from build123d import *

# Parameters (mm, degrees)
SKETCH1_W           = 28
SKETCH1_H           = 48
BOSS_EXTRUDE3_DEPTH = 60
SKETCH6_W           = 10
SKETCH6_H           = 35
CUT_EXTRUDE7_DEPTH  = 48
SKETCH7_W           = 25
SKETCH7_H           = 10
CUT_EXTRUDE8_DEPTH  = 48
SKETCH8_W           = 35
SKETCH8_H           = 28
BOSS_EXTRUDE4_DEPTH = 92
SKETCH9_R           = 6.25
CUT_EXTRUDE9_DEPTH  = 59
CUT_EXTRUDE12_DEPTH = 59
CUT_EXTRUDE13_DEPTH = 59
CUT_EXTRUDE18_DEPTH = 11


with BuildPart() as part:
    # Sketch1 → Boss-Extrude3 (new body)
    with BuildSketch(Plane.XY):
        with Locations((14, 24)):
            Rectangle(SKETCH1_W, SKETCH1_H)
    extrude(amount=BOSS_EXTRUDE3_DEPTH)

    # Sketch6 → Cut-Extrude7 (cut)
    with BuildSketch(Plane(origin=(0, 48, 0), x_dir=(1, 0, 0), z_dir=(0, 1, 0))):
        with Locations((23, -30)):
            Rectangle(SKETCH6_W, SKETCH6_H)
    extrude(amount=-CUT_EXTRUDE7_DEPTH, mode=Mode.SUBTRACT)

    # Sketch7 → Cut-Extrude8 (cut)
    with BuildSketch(Plane.ZY):
        with Locations((30, 43)):
            Rectangle(SKETCH7_W, SKETCH7_H)
    extrude(amount=-CUT_EXTRUDE8_DEPTH, mode=Mode.SUBTRACT)

    # Sketch8 → Boss-Extrude4 (add)
    with BuildSketch(Plane.ZY):
        with Locations((30, 14)):
            Rectangle(SKETCH8_W, SKETCH8_H)
    extrude(amount=BOSS_EXTRUDE4_DEPTH)

    # Sketch9 → Cut-Extrude9 (cut)
    with BuildSketch(Plane.XY.offset(47.5)):
        with Locations((-35, 14)):
            Circle(SKETCH9_R)
    extrude(amount=-CUT_EXTRUDE9_DEPTH, mode=Mode.SUBTRACT)

    # Sketch16 → Cut-Extrude12 (cut)
    with BuildSketch(Plane(origin=(0, 28, 0), x_dir=(1, 0, 0), z_dir=(0, 1, 0))):
        Polygon((-92, -30), (-73.408450704, -12.5), (-92, -12.5), align=None)
    extrude(amount=-CUT_EXTRUDE12_DEPTH, mode=Mode.SUBTRACT)

    # Sketch17 → Cut-Extrude13 (cut)
    with BuildSketch(Plane(origin=(0, 28, 0), x_dir=(1, 0, 0), z_dir=(0, 1, 0))):
        Polygon((-92, -30), (-92, -47.5), (-74.705382998, -47.5), align=None)
    extrude(amount=-CUT_EXTRUDE13_DEPTH, mode=Mode.SUBTRACT)

    # Sketch18 → Cut-Extrude18 (cut)
    with BuildSketch(Plane(origin=(0, 28, 0), x_dir=(1, 0, 0), z_dir=(0, 1, 0))):
        Polygon((-92, -30), (-78.644507081, -43.514096673), (-78.164969417, -16.977253409), align=None)
    extrude(amount=-CUT_EXTRUDE18_DEPTH, mode=Mode.SUBTRACT)


solid = part.part
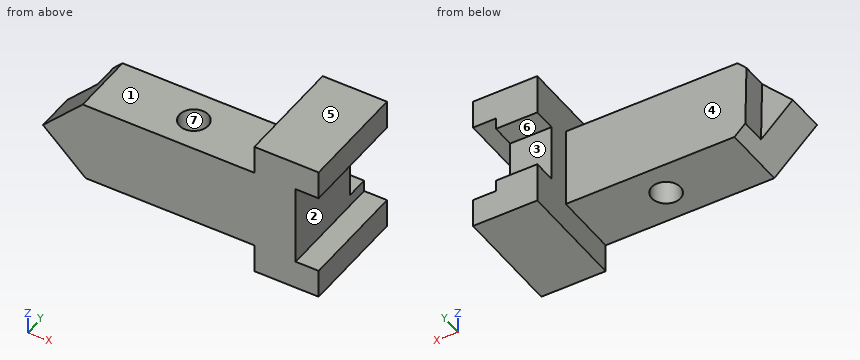
Could you check a few things on this model? Use its own coordinates, in mm. Face numbers are marked on the shaded views. A direction names the side the tool comes from. Give positions to 0.01 mm unless a question says otherwise; leave off trailing zeros. Order: outer loops, then holes, each group sorted by start corner. A loop starts at its lowest first (then second) coordinate and runs counter-clockwise, first axis right, second up. Notation, with made-up numbers: (39, 53) - (50, 53) arc R14 cw to (50, 65) - close; hole circle Ø1 at (-1, -15.5). An arc over 180 degrees is marked (long way). Return JSON: item names as keys, results as strings. Group by question number.
Q1. Suppose I cut it at C-C, the plane y = 23. Please give me the cut outline in (x, z), and give its area (3 significant figures).
Q2. Which directions (+Z, -Z, +X, -X, +Y, -Y) give clear straight access to the entire face, cutting with the end or side of a thin tool? Please do the marked faces 1, 2, 3 and 4.
Q3. Please list where these lines run through material, in increasing order: line 1 along Y through (x, z) = (-35, 38); line 2 along X through (y, z) = (31, 36); line 3 along Y through (x, z) = (-53, 35). Write a range as [from, to].
Q4. Will these pins go through, and if not, where does the flat tip stop? pin 1 Ø8.5 at (x, y) = (-53.5, 8) entering from -Z; pin 2 Ø12 at (y, z) = (25.5, 22.5) entering from +X; pin 3 Ø7 at (x, z) = (-87, 31) entering from +Y.
Q5. Suppose I cut it at B-B, the plane y = 45.5. Please give me the cut outline in (x, z).
Q6. Suppose I cut it at D-D, the plane z = 40.5. Please give me the cut outline in (x, y), and give its area (3 significant figures).
Q7. Thinking about a two-plate mould opening in Z: for the marked faces 5, 6 and 7, which applies, pulls with the +Z half, pulls with the -Z half, needs draft (parallel to the pull), parting line crosses it, or undercut?
Q8. Suppose I cut it at A-A, the plane x = -35. Please give me the cut outline in (y, z).
Resolved:
{
 "1": {"outline": "(-78.64, 43.51) - (-78.16, 16.98) - (-73.41, 12.5) - (0, 12.5) - (0, 0) - (28, 0) - (28, 12.5) - (18, 12.5) - (18, 47.5) - (28, 47.5) - (28, 60) - (0, 60) - (0, 47.5) - (-74.71, 47.5) - close", "area": "4,060 mm2"},
 "2": {"face 1": "+Z, -X, +Y, -Y", "face 2": "+X, +Y, -Y", "face 3": "+X, -X, +Y", "face 4": "+Z, -Z, -X, +Y"},
 "3": {"line 1": "y = [0, 7.75], [20.25, 28]", "line 2": "x = [0, 18]", "line 3": "y = [0, 28]"},
 "4": {"pin 1": "stops at z = 12.5", "pin 2": "stops at x = 18", "pin 3": "stops at y = 17"},
 "5": {"outline": "(0, 0) - (28, 0) - (28, 12.5) - (18, 12.5) - (18, 17.5) - (0, 17.5) - close; (0, 42.5) - (18, 42.5) - (18, 47.5) - (28, 47.5) - (28, 60) - (0, 60) - close"},
 "6": {"outline": "(-81.62, 0) - (18, 0) - (18, 38) - (0, 38) - (0, 28) - (-78.59, 28) - (-78.59, 17) - (-81.62, 17) - close; hole circle Ø12.5 at (-35, 14)", "area": "2,810 mm2"},
 "7": {"face 5": "pulls with the +Z half", "face 6": "undercut", "face 7": "needs draft"},
 "8": {"outline": "(0, 12.5) - (7.75, 12.5) - (7.75, 47.5) - (0, 47.5) - close; (20.25, 12.5) - (28, 12.5) - (28, 47.5) - (20.25, 47.5) - close"}
}
